```python
from build123d import *

# Parameters (mm, degrees)
PAD_DEPTH = 10


with BuildPart() as part:
    # Sketch → Pad (new body, symmetric)
    with BuildSketch(Plane.XZ):
        Polygon((-40, 0), (-20, 0), (-20, 40), (20, 40), (20, 0), (40, 0), (40, 60), (-40, 60), align=None)
    extrude(amount=PAD_DEPTH, both=True)


solid = part.part
```
Could you check a few things on this model? Use its own coordinates, in mm. A direction names the side the tool comes from. Coordinates: 2 decimals unless noted, no trailing zeros. Order: outer loops, then holes, each group sorted by start corner. A loop starts at its lowest first (then second) coordinate and runs counter-clockwise, first axis right, second up. Notation, with made-up numbers: M -34,78 L -30,78 A14 ccw -30,85 Z; hole C 78.25,53.25 d2. An arc over 180 degrees is marked long. Use a Markdown table: item, result. Add a question column.
Q1. I want a section at B-B on y = 4. List the corners of the cut face in (x, z) for me.
Q2. We'd pull the mould along X, two halves only. Please class faces 1 (the flat face through (40, 0, 30)), 2 (the flat face through (-40, 0, 30)), 3 (the flat face through (0, 0, 40)), 4 (the flat face through (-30, 0, 0)): pulls with the +X half, pulls with the -X half, needs draft (parallel to the pull), parting line crosses it, or undercut.
Q3. I want a section at C-C on x = -14. List the corners of the cut face in (y, z) for me, then the cut area to 3 significant figures.
Q4. If I drill on L1, parallel to X at y = -9, z = 29; L2, parallel to Z at x = -9, y = -5.5, over which ranges is the centre line in solid material (lowest first)?
Q5. I'm going to push a flat-ended pin straight in: pin 1 (8 mm diameter, centred on x = -15, y = -6, fed in from -Z). Where does the tip first touch, or does it pass through?
Q6. I want a section at A-A on z = 7.5. List the corners of the cut face in (x, y) for me, then the cut area to 3 significant figures.
Q7. Which directions (+Z, -Z, +X, -X, +Y, -Y) give clear straight access to the entire face, cutting with the end or side of a thin tool? Please do faces 5 (the flat face through (1, 0, 60)), 6 (the flat face through (20, 0, 20)).
Checked values:
| question | item | result |
|---|---|---|
| 1 | outline | M -40,0 L -20,0 L -20,40 L 20,40 L 20,0 L 40,0 L 40,60 L -40,60 Z |
| 2 | face 1 | pulls with the +X half |
| 2 | face 2 | pulls with the -X half |
| 2 | face 3 | undercut |
| 2 | face 4 | needs draft |
| 3 | outline | M -10,40 L 10,40 L 10,60 L -10,60 Z |
| 3 | area | 400 mm² |
| 4 | L1 | -40 to -20, 20 to 40 |
| 4 | L2 | 40 to 60 |
| 5 | pin 1 | z = 40 |
| 6 | outline | M -40,-10 L -20,-10 L -20,10 L -40,10 Z; M 20,-10 L 40,-10 L 40,10 L 20,10 Z |
| 6 | area | 800 mm² |
| 7 | face 5 | +Z, +X, -X, +Y, -Y |
| 7 | face 6 | -Z, +Y, -Y |
